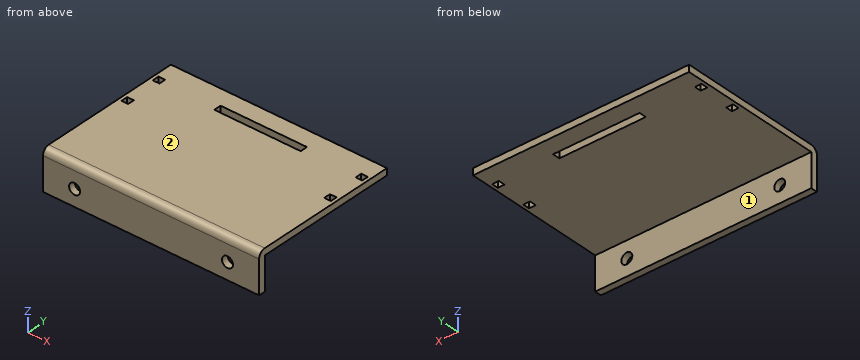
from build123d import *

# Parameters (mm, degrees)
SKETCH_1_W                   = 65
SKETCH_1_H                   = 45
SM_BASE_FLANGE_1_DEPTH       = 2
SM_START                     = -32.425287356
SM_EDGE_FLANGE_1_DEPTH       = 65
SM_EDGE_FLANGE_1_2_OUTLINE_W = 2
SM_EDGE_FLANGE_1_2_OUTLINE_H = 10
SM_EDGE_FLANGE_1_2_DEPTH     = 65
SKETCH_9_W                   = 2
SKETCH_9_H                   = 2
SKETCH_9_W_2                 = 26
SKETCH_9_H_2                 = 2.2
CUT_EXTRUDE_1_DEPTH          = 10
SKETCH_11_R                  = 1.65
CUT_EXTRUDE_3_DEPTH          = 10


# Read off the part's stored shape, not the designer's step: 边线-法兰1
# Sheet-metal steps are written as plain solids
with BuildPart() as part:
    # Sketch 1 → 基体-法兰1 (new body)
    with BuildSketch(Plane.XY):
        with Locations((0.074712644, -3.939027096)):
            Rectangle(SKETCH_1_W, SKETCH_1_H)
    extrude(amount=-SM_BASE_FLANGE_1_DEPTH)

    # 边线-法兰1 outline → 边线-法兰1 (cut)
    with BuildSketch(Plane.YZ.offset(SM_START)):
        with BuildLine():
            ThreePointArc((-26.439027096, -2), (-25.853240658, -0.585786437), (-24.439027096, 0))
            Line((-24.439027096, 0), (-26.439027096, 0))
            Line((-26.439027096, 0), (-26.439027096, -2))
        make_face()
    extrude(amount=SM_EDGE_FLANGE_1_DEPTH, mode=Mode.SUBTRACT)

    # Sm Edge Flange 1 2 outline → Sm Edge Flange 1 2 (add)
    with BuildSketch(Plane.YZ.offset(SM_START)):
        with Locations((-25.439027096, -7)):
            Rectangle(SM_EDGE_FLANGE_1_2_OUTLINE_W, SM_EDGE_FLANGE_1_2_OUTLINE_H)
    extrude(amount=SM_EDGE_FLANGE_1_2_DEPTH)

    # 草图9 → 切除-拉伸1 (cut)
    with BuildSketch(Plane.XY):
        with Locations((-30.425287356, 1)):
            Rectangle(SKETCH_9_W, SKETCH_9_H)
        with Locations((0.074712644, 12.1)):
            Rectangle(SKETCH_9_W_2, SKETCH_9_H_2)
        with Locations((30.574712644, 12)):
            Rectangle(SKETCH_9_W, SKETCH_9_H)
        with Locations((-30.425287356, 12)):
            Rectangle(SKETCH_9_W, SKETCH_9_H)
        with Locations((30.574712644, 1)):
            Rectangle(SKETCH_9_W, SKETCH_9_H)
    extrude(amount=-CUT_EXTRUDE_1_DEPTH, mode=Mode.SUBTRACT)

    # 草图11 → 切除-拉伸3 (cut)
    with BuildSketch(Plane(origin=(0, -24.439027096, 0), x_dir=(1, 0, 0), z_dir=(0, 1, 0))):
        with Locations(Location((-22.925287356, 7, 0), (0, 0, 270))):
            Circle(SKETCH_11_R)
        with Locations(Location((23.074712644, 7, 0), (0, 0, 90))):
            Circle(SKETCH_11_R)
    extrude(amount=-CUT_EXTRUDE_3_DEPTH, mode=Mode.SUBTRACT)


solid = part.part
For this review, take the finished solid that the model builds, in its own axes (mm). Face numbers are marked on the shaded views. A direction names the side the tool comes from. Coordinates: 2 decimals unless noted, no trailing zeros. Order: outer loops, then holes, each group sorted by start corner. A loop starts at its lowest first (then second) coordinate and runs counter-clockwise, first axis right, second up. Notation, with made-up numbers: (-13, -26) -> (-4, -26) arc R15 ccw to (-4, -21) -> close; hole circle Ø11 at (36.25, 28). An arc over 180 degrees is marked (long way). Return JSON: item names as keys, results as strings.
1. For line 1 (X direction, y = 1, z = -1.5); line 2 (X direction, y = -25, z = -7); line 3 (Y direction, x = -20, z = -10.75), list the stretches that pass through material, from the lowest coordinate up. Write a range as from..to.
Answer block:
{"line 1": "-32.43..-31.43, -29.43..29.57, 31.57..32.57", "line 2": "-32.43..-24.58, -21.28..21.42, 24.72..32.57", "line 3": "-26.44..-24.44"}
2. We need section D-D on z = -0.75. Write out the cut boundary in (x, y).
Answer block:
{"outline": "(-32.43, -26) -> (32.57, -26) -> (32.57, 18.56) -> (-32.43, 18.56) -> close; hole (-31.43, 0) -> (-29.43, 0) -> (-29.43, 2) -> (-31.43, 2) -> close; hole (-31.43, 11) -> (-29.43, 11) -> (-29.43, 13) -> (-31.43, 13) -> close; hole (-12.93, 11) -> (13.07, 11) -> (13.07, 13.2) -> (-12.93, 13.2) -> close; hole (29.57, 0) -> (31.57, 0) -> (31.57, 2) -> (29.57, 2) -> close; hole (29.57, 11) -> (31.57, 11) -> (31.57, 13) -> (29.57, 13) -> close"}
3. Machinability: for the marked faces 1 and 2, which of the approach directions +Z, -Z, +X, -X, +Y, -Y give a long, thin tool a straight path to every point of the face, cutting with its end or side? Answer none if there is none.
Answer block:
{"face 1": "-Z, +X, -X, +Y", "face 2": "+Z, +X, -X, +Y, -Y"}
4. We need section B-B on z = -7. Write out the cut boundary in (x, y).
Answer block:
{"outline": "(-32.43, -26.44) -> (-24.58, -26.44) -> (-24.58, -24.44) -> (-32.43, -24.44) -> close; (-21.28, -26.44) -> (21.42, -26.44) -> (21.42, -24.44) -> (-21.28, -24.44) -> close; (24.72, -26.44) -> (32.57, -26.44) -> (32.57, -24.44) -> (24.72, -24.44) -> close"}
5. We need section C-C on x = 19.5. Write out the cut boundary in (y, z).
Answer block:
{"outline": "(-26.44, -12) -> (-24.44, -12) -> (-24.44, -2) -> (18.56, -2) -> (18.56, 0) -> (-24.44, 0) arc R2 ccw to (-26.44, -2) -> close"}
6. For pin 1 Ø1 at (x, y) = (8.5, 11) entering from -Z; pin 2 Ø1.5 at (x, z) = (-21, -3.5) entering from +Y; pin 3 Ø0.6 at (x, z) = (-30, -1) entering from -Y; pin 4 Ø6 at (x, z) = (15.5, -3.5) entering from +Y, all flat-tipped, find the tip position at first contact; note any pin that passes through.
Answer block:
{"pin 1": "z = -2", "pin 2": "y = -24.44", "pin 3": "y = -26.31", "pin 4": "y = 18.56"}
7. We need section A-A on x = 7. Write out the cut boundary in (y, z), and give its area (3 significant figures).
Answer block:
{"outline": "(-26.44, -12) -> (-24.44, -12) -> (-24.44, -2) -> (11, -2) -> (11, 0) -> (-24.44, 0) arc R2 ccw to (-26.44, -2) -> close; (13.2, -2) -> (18.56, -2) -> (18.56, 0) -> (13.2, 0) -> close", "area": "105 mm²"}
